from build123d import *

# Parameters (mm, degrees)
SKETCH1_W                       = 75.438
SKETCH1_H                       = 12.7
BOSS_EXTRUDE1_DEPTH             = 6.35
CUT_EXTRUDE1_DEPTH              = 3.175
BOSS_EXTRUDE2_REACH             = 40.773
SKETCH3_W                       = 75.438
SKETCH3_H                       = 19.05
SKETCH3_W_2                     = 69.088
SKETCH3_H_2                     = 12.7
BOSS_EXTRUDE2_DIRECTION_2_REACH = 40.773
SKETCH4_W                       = 75.438
SKETCH4_H                       = 25.4
BOSS_EXTRUDE4_DEPTH             = 3.175
SKETCH7_W                       = 14.859
SKETCH7_H                       = 15.875
CUT_EXTRUDE3_DEPTH              = 47.460828512
SKETCH8_W                       = 3.175
SKETCH8_H                       = 15.875
CUT_EXTRUDE4_DEPTH              = 65.214043371
BOSS_EXTRUDE5_DEPTH             = 3.175
FILLET2_R                       = 1.905


with BuildPart() as part:
    # Sketch1 → Boss-Extrude1 (new body)
    with BuildSketch(Plane.XY):
        Rectangle(SKETCH1_W, SKETCH1_H)
    extrude(amount=BOSS_EXTRUDE1_DEPTH)

    # Sketch2 → Cut-Extrude1 (cut)
    with BuildSketch(Plane.XY.offset(6.35)):
        with BuildLine():
            Line((3.175, 5.129369479), (17.6006647, 2.498793645))
            ThreePointArc((17.6006647, 2.498793645), (19.685, 0), (17.6006647, -2.498793645))
            Line((17.6006647, -2.498793645), (3.175, -5.129369479))
            ThreePointArc((3.175, -5.129369479), (0, -6.0325), (-3.175, -5.129369479))
            Line((-3.175, -5.129369479), (-17.6006647, -2.498793645))
            ThreePointArc((-17.6006647, -2.498793645), (-19.685, 0), (-17.6006647, 2.498793645))
            Line((-17.6006647, 2.498793645), (-3.175, 5.129369479))
            ThreePointArc((-3.175, 5.129369479), (0, 6.0325), (3.175, 5.129369479))
        make_face()
    extrude(amount=-CUT_EXTRUDE1_DEPTH, mode=Mode.SUBTRACT)

    # Boss-Extrude2: up to this face of the body (flat: up to its plane)
    boss_extrude2_end = Plane(part.part.faces().sort_by_distance((0, 6.35, 3.175))[0])
    # Sketch3 → Boss-Extrude2 (add, up to the picked face)
    with BuildSketch(Plane(origin=(0, 0, 0), x_dir=(1, 0, 0), z_dir=(0, 1, 0)), mode=Mode.PRIVATE) as boss_extrude2_sk1:
        with Locations((0, 9.525)):
            Rectangle(SKETCH3_W, SKETCH3_H)
        with Locations((0, 9.525)):
            Rectangle(SKETCH3_W_2, SKETCH3_H_2, mode=Mode.SUBTRACT)
    boss_extrude2_tool1 = split(extrude(boss_extrude2_sk1.sketch, amount=BOSS_EXTRUDE2_REACH, mode=Mode.PRIVATE), bisect_by=boss_extrude2_end, keep=Keep.BOTH, mode=Mode.PRIVATE)
    add(boss_extrude2_tool1.solids().sort_by(Axis((0, 0, -0.778061), (0, 1, 0)))[0])

    # Boss-Extrude2 direction 2: up to this face of the body (flat: up to its plane)
    boss_extrude2_direction_2_end = Plane(part.part.faces().sort_by_distance((0, -6.35, 3.175))[0])
    # Sketch3 → Boss-Extrude2 direction 2 (add, up to the picked face)
    with BuildSketch(Plane(origin=(0, 0, 0), x_dir=(1, 0, 0), z_dir=(0, 1, 0)), mode=Mode.PRIVATE) as boss_extrude2_direction_2_sk1:
        with Locations((0, 9.525)):
            Rectangle(SKETCH3_W, SKETCH3_H)
        with Locations((0, 9.525)):
            Rectangle(SKETCH3_W_2, SKETCH3_H_2, mode=Mode.SUBTRACT)
    boss_extrude2_direction_2_tool1 = split(extrude(boss_extrude2_direction_2_sk1.sketch, amount=-BOSS_EXTRUDE2_DIRECTION_2_REACH, mode=Mode.PRIVATE), bisect_by=boss_extrude2_direction_2_end, keep=Keep.BOTH, mode=Mode.PRIVATE)
    add(boss_extrude2_direction_2_tool1.solids().sort_by(Axis((0, 0, -0.778061), (0, -1, 0)))[0])

    # Sketch4 → Boss-Extrude4 (add)
    with BuildSketch(Plane(origin=(0, 6.35, 0), x_dir=(1, 0, 0), z_dir=(0, 1, 0))):
        with Locations((0, 6.35)):
            Rectangle(SKETCH4_W, SKETCH4_H)
    extrude(amount=BOSS_EXTRUDE4_DEPTH)

    # Sketch7 → Cut-Extrude3 (cut, through all)
    with BuildSketch(Plane.XY.offset(6.35)):
        with Locations((30.2895, 1.5875)):
            Rectangle(SKETCH7_W, SKETCH7_H)
    extrude(amount=-CUT_EXTRUDE3_DEPTH, mode=Mode.SUBTRACT)

    # Sketch8 → Cut-Extrude4 (cut, through all)
    with BuildSketch(Plane(origin=(22.86, 0, 0), x_dir=(0, 0, -1), z_dir=(1, 0, 0))):
        with Locations((17.4625, 1.5875)):
            Rectangle(SKETCH8_W, SKETCH8_H)
    extrude(amount=-CUT_EXTRUDE4_DEPTH, mode=Mode.SUBTRACT)

    # Sketch9 → Boss-Extrude5 (add)
    with BuildSketch(Plane(origin=(0, 0, -15.875), x_dir=(-1, 0, 0), z_dir=(0, 0, -1))):
        Polygon((34.544, 6.35), (34.544, -6.35), (37.719, -6.35), (37.719, 9.525), (-22.86, 9.525), (-22.86, 6.35), align=None)
    extrude(amount=BOSS_EXTRUDE5_DEPTH)

    # Fillet2
    # the kernel refuses this fillet: 1.905 mm, written as the material it adds along each edge
    with BuildSketch(Plane(origin=(-34.544, 6.35, 1.5875), x_dir=(0, -1, 0), z_dir=(0, 0, -1))) as fillet2_piece_1:
        with BuildLine():
            CenterArc((FILLET2_R, -FILLET2_R), FILLET2_R, 90, 90)
            Line((0, -FILLET2_R), (0, 0))
            Line((0, 0), (FILLET2_R, 0))
        make_face()
    extrude(amount=20.6375)
    # the kernel refuses this fillet: 1.905 mm, written as the material it takes off along each edge
    with BuildSketch(Plane(origin=(-37.719, 9.525, 11.1125), x_dir=(0, -1, 0), z_dir=(0, 0, -1)), Plane(origin=(-37.719, -6.35, 11.1125), x_dir=(1, 0, 0), z_dir=(0, 0, -1))) as fillet2_2_piece_1:
        with BuildLine():
            CenterArc((FILLET2_R, -FILLET2_R), FILLET2_R, 90, 90)
            Line((0, -FILLET2_R), (0, 0))
            Line((0, 0), (FILLET2_R, 0))
        make_face()
    extrude(amount=34.925, mode=Mode.SUBTRACT)
    with BuildSketch(Plane(origin=(-34.544, -6.35, -3.175), x_dir=(0, 1, 0), z_dir=(0, 0, -1))) as fillet2_2_piece_2:
        with BuildLine():
            CenterArc((FILLET2_R, -FILLET2_R), FILLET2_R, 90, 90)
            Line((0, -FILLET2_R), (0, 0))
            Line((0, 0), (FILLET2_R, 0))
        make_face()
    extrude(amount=20.6375, mode=Mode.SUBTRACT)
    with BuildSketch(Plane(origin=(22.86, 6.35, -23.8125), x_dir=(0, 1, 0), z_dir=(0, 0, 1))) as fillet2_2_piece_3:
        with BuildLine():
            CenterArc((FILLET2_R, FILLET2_R), FILLET2_R, 180, 90)
            Line((0, FILLET2_R), (0, 0))
            Line((0, 0), (FILLET2_R, 0))
        make_face()
    extrude(amount=20.6375, mode=Mode.SUBTRACT)
    with BuildSketch(Plane(origin=(22.86, 9.525, -23.8125), x_dir=(-1, 0, 0), z_dir=(0, 0, 1))) as fillet2_2_piece_4:
        with BuildLine():
            CenterArc((FILLET2_R, FILLET2_R), FILLET2_R, 180, 90)
            Line((0, FILLET2_R), (0, 0))
            Line((0, 0), (FILLET2_R, 0))
        make_face()
    extrude(amount=34.925, mode=Mode.SUBTRACT)
    with BuildSketch(Plane(origin=(22.86, -6.35, 11.1125), x_dir=(-1, 0, 0), z_dir=(0, 0, -1))) as fillet2_2_piece_5:
        with BuildLine():
            CenterArc((FILLET2_R, FILLET2_R), FILLET2_R, 180, 90)
            Line((0, FILLET2_R), (0, 0))
            Line((0, 0), (FILLET2_R, 0))
        make_face()
    extrude(amount=19.05, mode=Mode.SUBTRACT)


solid = part.part
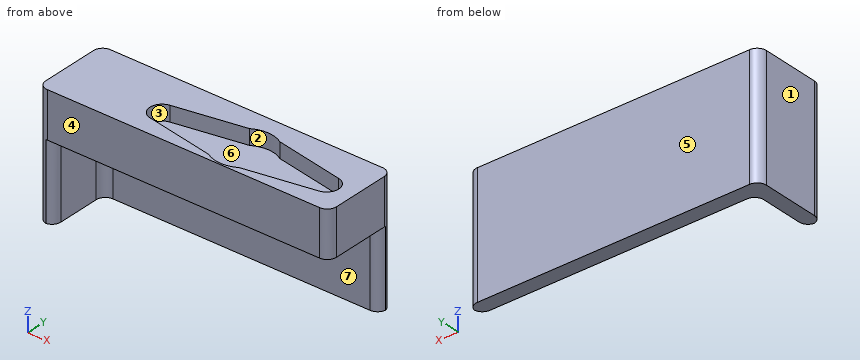
Geometry check sheet. Reference: the model listing, model coordinates, mm. Face numbers are marked on the shaded views. A direction names the side the tool comes from. Give positions to 0.01 mm unless a question says otherwise; leave off trailing zeros. Loops run counter-clockwise (first coordinate to the right, second up) from the corner with the lowest first, then second, coordinate; pieces in that order, holes last. Notation, with made-up numbers: (12.5, 15.25) -> (16.5, 15.25) arc R31 cw to (16.5, 43.25) -> close; hole circle Ø5 at (80, 1.25). An arc over 180 degrees is marked (long way). Answer in a Markdown table with one row per item. Add a question column.
1) Set-up check for the marked faces 5, 6 and 7: record each of +Z, -Z, +X, -X, +Y, -Y from which the full face is reachable in a straight line by a thin tool's end or side.
2) Cross-section at A-A on y = 0. Record the boundary of the cut face in (x, z) (3 decimals).
3) Material ranges on probe 1 along Y at (x, z) = (20, -9) (3 decimals); probe 2 along Z at (x, y) = (16, 1.75) (3 decimals); probe 3 along Z at (x, y) = (-34, 3.75) (3 decimals), recorded low to high. Write a range as from..to.
4) Gauge pin test, flat ends, axial feed: P1, Ø3.5, axis at x = 4.5, y = -1, coming from the +Z side (3 decimals); P2, Ø4, axis at x = -6, y = 1.5, coming from the -Z side (3 decimals); P3, Ø6, axis at y = -3, z = -9, coming from the +X side. Record the tip position at first contact, or that the pin passes through.
5) Cross-section at C-C on x = -30. Record the boundary of the cut face in (y, z) (3 decimals).
6) Draft check along Y on the marked faces 1, 2, 3 and 4. Enter one of: pulls with the +Y half, pulls with the -Y half, needs draft (parallel to the pull), parting line crosses it, or undercut.
Outcome:
| question | item | result |
|---|---|---|
| 1 | face 5 | +Z, -Z, +X, -X, +Y |
| 1 | face 6 | +Z |
| 1 | face 7 | -Z, +X, -Y |
| 2 | outline | (-37.719, -19.05) -> (-34.544, -19.05) -> (-34.544, -3.175) -> (22.86, -3.175) -> (22.86, 6.35) -> (19.685, 6.35) -> (19.685, 3.175) -> (-19.685, 3.175) -> (-19.685, 6.35) -> (-37.719, 6.35) -> close |
| 3 | probe 1 | y = 6.35..9.525 |
| 3 | probe 2 | z = -3.175..3.175 |
| 3 | probe 3 | z = -3.175..6.35 |
| 4 | P1 | stops at z = 3.175 |
| 4 | P2 | stops at z = -3.175 |
| 4 | P3 | stops at x = -34.54 |
| 5 | outline | (-6.35, -3.175) -> (6.35, -3.175) -> (6.35, -19.05) -> (9.525, -19.05) -> (9.525, 6.35) -> (-6.35, 6.35) -> close |
| 6 | face 1 | needs draft |
| 6 | face 2 | undercut |
| 6 | face 3 | undercut |
| 6 | face 4 | pulls with the -Y half |
